```python
from build123d import *

# Parameters (mm, degrees)
F1_DEPTH = 19.05
F2_R     = 12.7
F3_R     = 6.35
F4_R     = 6.35


with BuildPart() as f1:
    # F0 (on Right) → F1 (new body)
    with BuildSketch(Plane.YZ):
        Polygon((-495.3, -771.525), (495.3, -771.525), (495.3, 771.525), (495.3, 974.725), (-38.1, 974.725), (-38.1, 771.525), (-495.3, 771.525), align=None)
    extrude(amount=F1_DEPTH)

    # F2
    f2_edges = [f1.edges().sort_by_distance(p)[0] for p in [
        (19.05, -266.7, 771.525),
    ]]
    fillet(f2_edges, radius=F2_R)

    # F3
    f3_edges = [f1.edges().sort_by_distance(p)[0] for p in [
        (19.05, 228.6, 974.725),
        (0, 228.6, 974.725),
    ]]
    fillet(f3_edges, radius=F3_R)

    # F4
    f4_edges = [f1.edges().sort_by_distance(p)[0] for p in [
        (19.05, -38.1, 869.95),
        (0, -38.1, 869.95),
    ]]
    fillet(f4_edges, radius=F4_R)


solid = f1.part
```
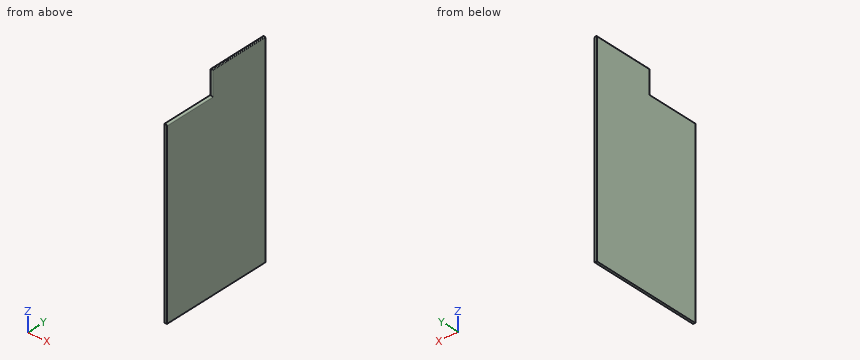
Build history of the part. All positions in model axes, mm. Round coordinates to 2 decimals unless told otherwise and drop trailing zeros. Write each loop counter-clockwise with the first axis right and the second up, starting at its lowest first coordinate (ties: lowest second). Pieces come first, ordered by that corner, then holes.
1) Band-saw the part on A-A, the plane y = -324.5. List the corners of the cut face in (x, z) (3 decimals).
2) Band-saw the part on C-C, the plane x = 16. List the corners of the cut face in (y, z) (3 decimals), and give its area (3 significant figures).
3) Band-saw the part on B-B, the plane z = 824.5. List the corners of the cut face in (x, y).
4) Pin check, flat tips, straight feed: pin 1 (2 mm diameter, centred on x = 3.5, y = -377, fed in from +Z) (3 decimals); pin 2 (7 mm diameter, centred on x = 10.5, z = 837.5, fed in from -Y). Stop position of each tip, or through.
5) Drill centre lines: probe 1 along Z at (x, y) = (7.25, -170.5) (3 decimals); probe 2 along Z at (x, y) = (7.75, -43) (3 decimals); probe 3 along Y at (x, z) = (15.25, 856). Where is each one in solid material? Low to high.
Ans:
1. outline: (0, -771.525) - (19.05, -771.525) - (19.05, 758.825) arc R12.7 ccw to (6.35, 771.525) - (0, 771.525) - close
2. outline: (-495.3, -771.525) - (495.3, -771.525) - (495.3, 973.8) - (-31.75, 973.8) arc R5.425 ccw to (-37.175, 968.375) - (-37.175, 767.081) - (-495.3, 767.081) - close
2. area: 1,630,000 mm2
3. outline: (0, -31.75) arc R6.35 ccw to (6.35, -38.1) - (12.7, -38.1) arc R6.35 ccw to (19.05, -31.75) - (19.05, 495.3) - (0, 495.3) - close
4. pin 1: stops at z = 771.525
4. pin 2: stops at y = -38.1
5. probe 1: z = -771.525 to 771.493
5. probe 2: z = -771.525 to 771.448
5. probe 3: y = -37.57 to 495.3
